```python
from build123d import *

# Parameters (mm, degrees)
BOSS_EXTRUDE3_DEPTH = 19.05


with BuildPart() as part:
    # Sketch3 → Boss-Extrude3 (new body)
    with BuildSketch(Plane(origin=(0, 0, 0), x_dir=(1, 0, 0), z_dir=(0, 1, 0))):
        Polygon((-77.838783367, 0), (-75.186491142, -20.146159583), (-67.410363796, -38.919391684), (-55.040331558, -55.040331558), (-38.919391684, -67.410363796), (-20.146159583, -75.186491142), (0, -77.838783367), (20.146159583, -75.186491142), (38.919391684, -67.410363796), (55.040331558, -55.040331558), (67.410363796, -38.919391684), (75.186491142, -20.146159583), (77.838783367, 0), (75.186491142, 20.146159583), (67.410363796, 38.919391684), (55.040331558, 55.040331558), (38.919391684, 67.410363796), (20.146159583, 75.186491142), (0, 77.838783367), (-20.146159583, 75.186491142), (-38.919391684, 67.410363796), (-55.040331558, 55.040331558), (-67.410363796, 38.919391684), (-75.186491142, 20.146159583), align=None)
        Polygon((-43.252896309, 0), (-41.779089607, -11.194673321), (-37.458106991, -21.626448155), (-30.584416286, -30.584416286), (-21.626448155, -37.458106991), (-11.194673321, -41.779089607), (0, -43.252896309), (11.194673321, -41.779089607), (21.626448155, -37.458106991), (30.584416286, -30.584416286), (37.458106991, -21.626448155), (41.779089607, -11.194673321), (43.252896309, 0), (41.779089607, 11.194673321), (37.458106991, 21.626448155), (30.584416286, 30.584416286), (21.626448155, 37.458106991), (11.194673321, 41.779089607), (0, 43.252896309), (-11.194673321, 41.779089607), (-21.626448155, 37.458106991), (-30.584416286, 30.584416286), (-37.458106991, 21.626448155), (-41.779089607, 11.194673321), align=None, mode=Mode.SUBTRACT)
    extrude(amount=BOSS_EXTRUDE3_DEPTH)


solid = part.part
```
Work out the finished part from the listing and answer in its coordinate system (mm). A direction names the side the tool comes from. Coordinates: 2 decimals unless noted, no trailing zeros. Write each loop counter-clockwise with the first axis right and the second up, starting at its lowest first coordinate (ties: lowest second). Pieces come first, ordered by that corner, then holes.
Q1. Which of the six approach directions +Z, -Z, +X, -X, +Y, -Y give full straight-line access (tool end or side, diameter ignored) to faces 1 (the face through (-71.353, 9.392, 29.401)), 2 (the face through (42.506, 9.392, 5.676))?
Q2. A cutting plane is placed at D-D, the plane x = -50. Give the vertices of the cut face in (y, z), then the cut area to 3 significant figures.
Q3. A cutting plane is placed at B-B, the plane z = 13.5. Give the vertices of the cut face in (x, y), then the cut area to 3 significant figures.
Q4. Determine the mould class of faces 3 (the face through (10.214, 9.392, -76.494)), 4 (the face through (71.244, 9.392, 29.664)), 5 (the face through (42.526, 9.392, -5.519)), 6 (the face through (16.338, 9.392, 39.649)) for opening direction Z: released by +Z, released by -Z, zero draft, split by the parting line, or undercut.
Q5. A cutting plane is placed at A-A, the plane x = -4.5. Give the vertices of the cut face in (y, z), then the cut area to 3 significant figures.
Q6. Each of these flat-tipped pins is pushed along its axis until it touches: pin 1 Ø1.5 at (y, z) = (7.5, -26.5) entering from +X; pin 2 Ø1.5 at (x, y) = (33.5, 14) entering from +Z; pin 3 Ø3 at (y, z) = (2.5, -4) entering from -X; pin 4 Ø4 at (x, z) = (-44, 38) entering from -Y. Where does it stop, or does it pass through?
Q7. A cutting plane is placed at C-C, the plane z = 51. Give the vertices of the cut face in (x, y).
Q8. Find the intervals of material crossed by line 1 (Z direction, x = 8, y = 7.75); line 2 (Z direction, x = 22.5, y = 1.25); line 3 (X direction, y = 1.25, z = 6), in increasing order.
Findings below:
1. face 1: +Z, -X, +Y, -Y
1. face 2: +Y, -Y
2. outline: (0, -58.91) - (19.05, -58.91) - (19.05, 58.91) - (0, 58.91) - close
2. area: 2,240 mm2
3. outline: (-76.06, 0) - (-40.82, 0) - (-40.82, 19.05) - (-76.06, 19.05) - close; (40.82, 0) - (76.06, 0) - (76.06, 19.05) - (40.82, 19.05) - close
3. area: 1,340 mm2
4. face 3: released by -Z
4. face 4: released by +Z
4. face 5: undercut
4. face 6: undercut
5. outline: (0, -77.25) - (19.05, -77.25) - (19.05, -42.66) - (0, -42.66) - close; (0, 42.66) - (19.05, 42.66) - (19.05, 77.25) - (0, 77.25) - close
5. area: 1,320 mm2
6. pin 1: stops at x = 72.87
6. pin 2: stops at z = 69.97
6. pin 3: stops at x = -77.51
6. pin 4: stops at y = 0
7. outline: (-58.14, 0) - (58.14, 0) - (58.14, 19.05) - (-58.14, 19.05) - close
8. line 1: z = -76.79 to -42.2, 42.2 to 76.79
8. line 2: z = -74.21 to -36.79, 36.79 to 74.21
8. line 3: x = -77.05 to -42.46, 42.46 to 77.05
